from build123d import *

# Parameters (mm, degrees)
F0_W      = 7
F0_H      = 7
F1_DEPTH  = 10
F2_W      = 7
F2_H      = 7
F3_DEPTH  = 30
F4_W      = 52.0183453336
F4_H      = 10
F5_DEPTH  = 5
F6_W      = 52.0183453336
F6_H      = 5
F7_DEPTH  = 16
F8_W      = 36
F8_H      = 16
F9_DEPTH  = 25
F10_DEPTH = 25
F11_DEPTH = 10


with BuildPart() as f1:
    # F0 (on Top) → F1 (new body)
    with BuildSketch(Plane.XY):
        Polygon((65.8497434995, 2.3738544621), (65.8497434995, 22.3738544621), (55.8497434995, 22.3738544621), (48.8497434995, 22.3738544621), (12.8497434995, 22.3738544621), (5.8497434995, 22.3738544621), (-4.1502565005, 22.3738544621), (-4.1502565005, 2.3738544621), align=None)
        with Locations((52.3497434995, 25.8738544621)):
            Rectangle(F0_W, F0_H)
        with Locations((9.3497434995, 25.8738544621)):
            Rectangle(F0_W, F0_H)
    extrude(amount=F1_DEPTH)

    # F2 (on face) → F3 (join)
    with BuildSketch(Plane.XY.offset(10)):
        with Locations((9.3497434995, 25.8738544621)):
            Rectangle(F2_W, F2_H)
        with Locations((52.3497434995, 25.8738544621)):
            Rectangle(F2_W, F2_H)
    extrude(amount=F3_DEPTH)

    # F4 (on face) → F5 (join)
    with BuildSketch(Plane.XZ.offset(-2.3738544621)):
        with Locations((30.9461015277, 5)):
            Rectangle(F4_W, F4_H)
    extrude(amount=F5_DEPTH)

    # F6 (on face) → F7 (join)
    with BuildSketch(Plane.XY.offset(10)):
        with Locations((30.9461015277, -0.1261455379)):
            Rectangle(F6_W, F6_H)
    extrude(amount=F7_DEPTH)

    # F8 (on face) → F9 (cut)
    with BuildSketch(Plane.XZ.offset(2.6261455379)):
        with Locations((30.8497434995, 18)):
            Rectangle(F8_W, F8_H)
    extrude(amount=-F9_DEPTH, mode=Mode.SUBTRACT)

    # F8 (on face) → F10 (cut)
    with BuildSketch(Plane.XZ.offset(2.6261455379)):
        with Locations((30.8497434995, 18)):
            Rectangle(F8_W, F8_H)
    extrude(amount=-F10_DEPTH, mode=Mode.SUBTRACT)

    # F11 (add): a face of the model
    f11_faces = [f1.faces().sort_by_distance(p)[0] for p in [
        (30.8639986862, 11.2771275086, 0),
    ]]
    extrude(f11_faces, amount=F11_DEPTH)


solid = f1.part
The model under review builds one solid part; all positions refer to its coordinate system, in mm. A direction names the side the tool comes from. Coordinates: 2 decimals unless noted, no trailing zeros. Write each loop counter-clockwise with the first axis right and the second up, starting at its lowest first coordinate (ties: lowest second). Pieces come first, ordered by that corner, then holes. Notation, with made-up numbers: (4.25, -8) - (50.25, -8) arc R28 ccw to (50.25, 17) - close; hole circle Ø4 at (72, 63). An arc over 180 degrees is marked (long way). Answer as a JSON object with one key per item and string values. Group by question number.
1. Add section A-A (z = 33.5). Give the boundary of the cut face in (x, y).
2. Mouldability with a two-part tool opening along Y and no side actions: class faces 5 (the face through (9, 2.374, 18)), 6 (the face through (9, 29.374, 15)), 7 (the face through (5.85, 26, 15)) as pulls with the +Y half, pulls with the -Y half, needs draft (parallel to the pull), parting line crosses it, or undercut.
3. Add section C-C (z = 22). Give the boundary of the cut face in (x, y), plus the area to 3 significant figures.
4. To check wall thickness, follow probe 1 along X at (y, z) = (25, 18.5); probe 2 along Y at (x, z) = (5, -7); probe 3 along Z at (x, y) = (37, -1). State the ranges of each line that lie inside material, in increasing order.
5. Clearance check with flat-ended pins moving along their axes: pin 1 Ø2 at (y, z) = (25.5, 14) entering from -X; pin 2 Ø16 at (x, z) = (22, 2.5) entering from +Y; pin 3 Ø6 at (x, y) = (52.5, 16) entering from +Z. State where each tip first meets the part, or that it passes through.
6. Add section B-B (y = 25). Give the boundary of the cut face in (x, z).
7. Add section D-D (x = 12). Give the boundary of the cut face in (y, z).
8. Machinability: for faces 1 (the face through (61, 22.374, 0)), 2 (the face through (9, 0, 26)), 3 (the face through (48.85, 0, 18)), 4 (the face through (61, 2.374, 0)), which of the approach directions +Z, -Z, +X, -X, +Y, -Y give a long, thin tool a straight path to every point of the face, cutting with its end or side? Answer none if there is none.
Findings:
{
 "1": {"outline": "(5.85, 22.37) - (12.85, 22.37) - (12.85, 29.37) - (5.85, 29.37) - close; (48.85, 22.37) - (55.85, 22.37) - (55.85, 29.37) - (48.85, 29.37) - close"},
 "2": {"face 5": "undercut", "face 6": "pulls with the +Y half", "face 7": "needs draft"},
 "3": {"outline": "(4.94, -2.63) - (12.85, -2.63) - (12.85, 2.37) - (4.94, 2.37) - close; (5.85, 22.37) - (12.85, 22.37) - (12.85, 29.37) - (5.85, 29.37) - close; (48.85, -2.63) - (56.96, -2.63) - (56.96, 2.37) - (48.85, 2.37) - close; (48.85, 22.37) - (55.85, 22.37) - (55.85, 29.37) - (48.85, 29.37) - close", "area": "178 mm²"},
 "4": {"probe 1": "5.85 to 12.85, 48.85 to 55.85", "probe 2": "-2.63 to 22.37", "probe 3": "-10 to 10"},
 "5": {"pin 1": "x = 5.85", "pin 2": "y = 22.37", "pin 3": "z = 10"},
 "6": {"outline": "(5.85, -10) - (12.85, -10) - (12.85, 40) - (5.85, 40) - close; (48.85, -10) - (55.85, -10) - (55.85, 40) - (48.85, 40) - close"},
 "7": {"outline": "(-2.63, -10) - (29.37, -10) - (29.37, 40) - (22.37, 40) - (22.37, 10) - (2.37, 10) - (2.37, 26) - (-2.63, 26) - close"},
 "8": {"face 1": "+Z, -Z, +X, +Y", "face 2": "+Z, +X, -X, -Y", "face 3": "+Z, +Y, -Y", "face 4": "+Z, -Z, +X, -Y"}
}
